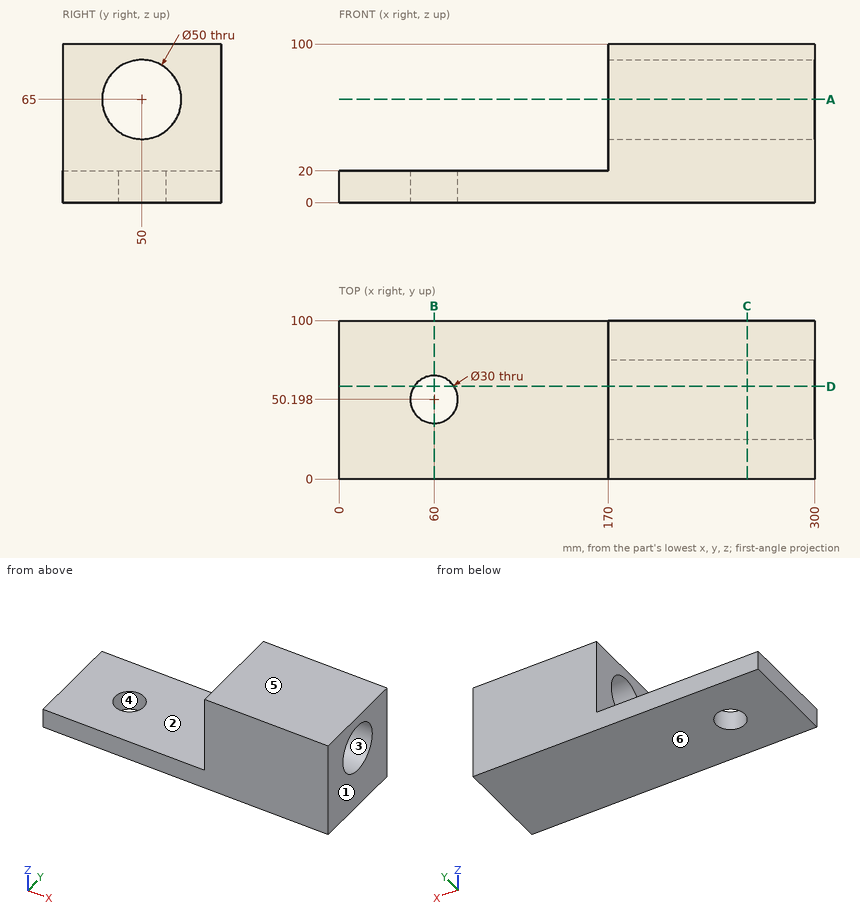
Study the drawing (mm; zero at the part's minimum x, y, z) and answer. A direction names the side the tool comes from. Coordinates: 2 decimals unless noted, no trailing zeros. Write each loop counter-clockwise with the first axis right and the second up, starting at its lowest first coordinate (ties: lowest second). Pieces come first, ordered by that corner, then holes. Notation, with made-up numbers: (44, -11) - (87, -11) arc R8 cw to (87, 4) - close; hole circle Ø3 at (37.25, -1.5). An arc over 180 degrees is marked (long way). One line per question, with ' | ' between items.
1) The mould has two halves that part along Z. Classify the marked faces 3, 4, 5 and 6: +Z half, -Z half, draft (parallel to the pull), parting line (faces both ways), or undercut.
Checks:
face 3: undercut | face 4: draft | face 5: +Z half | face 6: -Z half
2) Find section C-C, the plane x = 257.5. Determine the outline of the cut face in (y, z), and give its area (3 significant figures).
Checks:
outline: (0, 0) - (100, 0) - (100, 100) - (0, 100) - close; hole circle Ø50 at (50, 65) | area: 8,040 mm2
3) For the marked faces 1 and 2, determine the directions among +Z, -Z, +X, -X, +Y, -Y from which every point of the face is accessible in a straight line to the end or side of a thin tool.
Checks:
face 1: +Z, -Z, +X, +Y, -Y | face 2: +Z, -X, +Y, -Y
4) Find section A-A, the plane z = 65. Determine the outline of the cut face in (x, y), and give its area (3 significant figures).
Checks:
outline: (170, 0) - (300, 0) - (300, 25) - (170, 25) - close; (170, 75) - (300, 75) - (300, 100) - (170, 100) - close | area: 6,500 mm2
5) Consider probe 1 along Y at (x, z) = (60, 10); probe 2 along Z at (x, y) = (226, 51); probe 3 along Z at (x, y) = (34, 64.5). Determine where each line is inside the solid, lowest interval first. Write a range as [from, to].
Checks:
probe 1: [0, 35.2], [65.2, 100] | probe 2: [0, 40.02], [89.98, 100] | probe 3: [0, 20]
6) Find section B-B, the plane x = 60. Determine the outline of the cut face in (y, z), and give its area (3 significant figures).
Checks:
outline: (0, 0) - (35.2, 0) - (35.2, 20) - (0, 20) - close; (65.2, 0) - (100, 0) - (100, 20) - (65.2, 20) - close | area: 1,400 mm2
7) Flat-ended cylindrical pins translate along their axes: P1, Ø3, axis at x = 119.5, y = 63.5, coming from the +Z side; P2, Ø1.5, axis at x = 189.5, z = 62.5, coming from the -Y side. Find the tip coordinate at first contact, or state that the pin passes through.
Checks:
P1: z = 20 | P2: y = 0
8) Find section D-D, the plane y = 58.5. Determine the outline of the cut face in (x, z).
Checks:
outline: (0, 0) - (47.51, 0) - (47.51, 20) - (0, 20) - close; (72.49, 0) - (300, 0) - (300, 41.49) - (170, 41.49) - (170, 20) - (72.49, 20) - close; (170, 88.51) - (300, 88.51) - (300, 100) - (170, 100) - close
